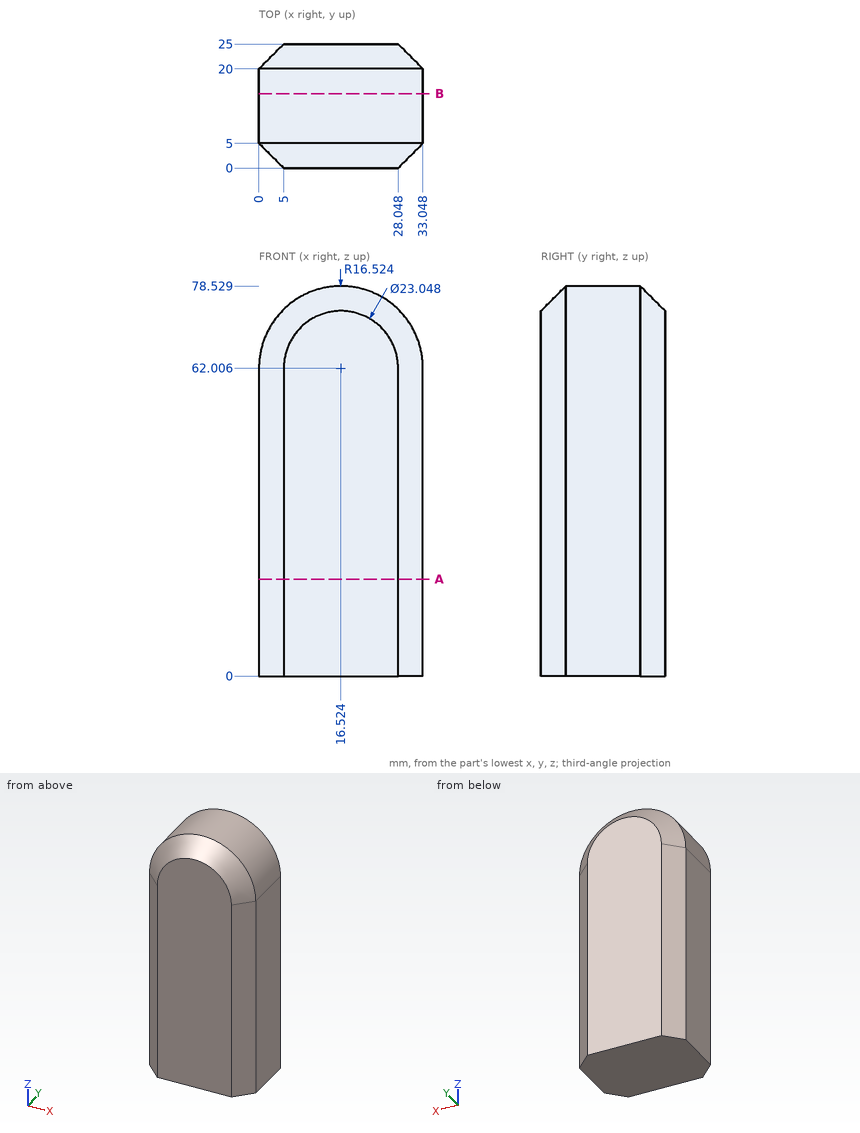
Job drawing, mm, ordinate dimensions from the low corner. One solid piece. Coordinates: 2 decimals unless noted, no trailing zeros. Write each loop counter-clockwise with the first axis right and the second up, starting at its lowest first coordinate (ties: lowest second). Pieces come first, ordered by that corner, then holes. Notation, with made-up numbers: M 1,27 L 30,27 A18 cw 30,32 Z; hole C -3.75,33.5 d6. An arc over 180 degrees is marked long. Answer as a JSON object with one key per item and string values. Group by question number.
1) Saw through at B-B (y = 15). Write the cut outline in (x, z) (1 decimal).
2) Pin check, flat tips, straight feed: pin 1 Ø2 at (x, y) = (10, 16) entering from +Z; pin 2 Ø5 at (x, y) = (26, 12) entering from +Z (1 decimal); pin 3 Ø1.5 at (x, y) = (28, 19.5) entering from +Z (1 decimal). Stop position of each tip, or through.
3) Wall check: line 1 (Z direction, x = 16, y = 6.75); line 2 (X direction, y = 17.5, z = 62.5); line 3 (Y direction, x = 3, z = 26.5). Give the ranges that are in metal, low to high. Write a range as from..to.
4) Saw through at A-A (z = 19.5). Write the cut outline in (x, y).
Values follow:
{
 "1": {"outline": "M 0,0 L 33,0 L 33,62 A16.5 ccw 0,62 Z"},
 "2": {"pin 1": "stops at z = 77.58", "pin 2": "stops at z = 77", "pin 3": "stops at z = 74.6"},
 "3": {"line 1": "z = 0..78.52", "line 2": "x = 0.01..33.04", "line 3": "y = 2..23"},
 "4": {"outline": "M 0,5 L 5,0 L 28.05,0 L 33.05,5 L 33.05,20 L 28.05,25 L 5,25 L 0,20 Z"}
}
